Source: three-view drawing plus pictorial views. Frame: mm from the lowest corner of the part. A direction names the side the tool comes from. Give positions to 0.01 mm unless a question says otherwise; leave off trailing zeros. Write each loop counter-clockwise with the first axis right and the second up, starting at its lowest first coordinate (ties: lowest second). Pieces come first, ordered by that corner, then holes. Notation, with made-up numbers: M 57.5,29.25 L 66.5,29.25 A23 ccw 66.5,41.25 Z; hole C -13.75,11 d7. An arc over 180 degrees is marked long. One line per question, with ' | ' between items.
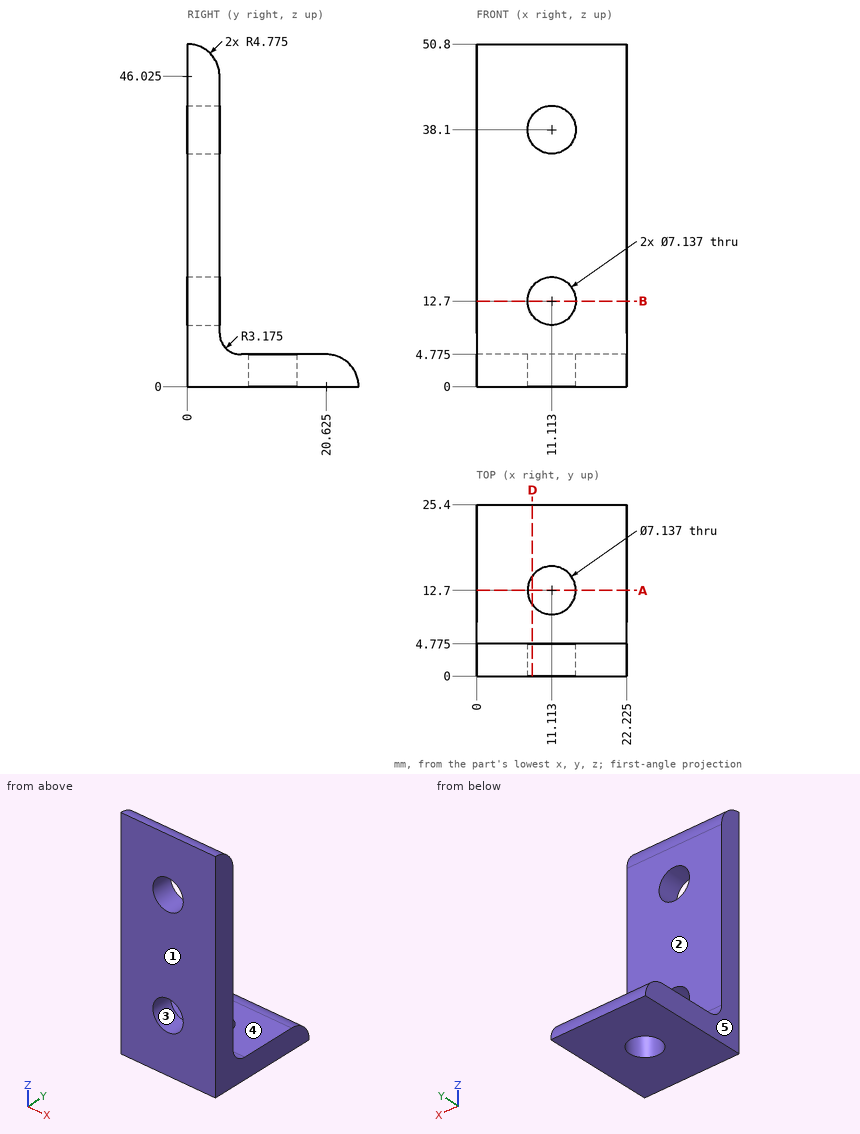
(1) Cut plane D-D, the plane x = 8.25. Count the separate pieces of the cut face and the enclosed holes in it.
Working result:
separate pieces: 4 | enclosed holes: 0
(2) Draft query along X for the marked faces 3, 4 and 5. Return one class per face: released by +X, released by -X, zero draft, split by the parting line, or undercut.
Working result:
face 3: undercut | face 4: zero draft | face 5: released by -X
(3) Set-up query: the marked faces 1 and 2. Return all of +Z, -Z, +X, -X, +Y, -Y with unobstructed straight access to the full face (end or side cutting, diameter ignored); none if empty.
Working result:
face 1: +Z, -Z, +X, -X, -Y | face 2: +Z, +X, -X, +Y
(4) Cut plane A-A, the plane y = 12.7. Return loops of the section in (x, z) (1 decimal).
Working result:
outline: M 0,0 L 7.5,0 L 7.5,4.8 L 0,4.8 Z; M 14.7,0 L 22.2,0 L 22.2,4.8 L 14.7,4.8 Z
(5) First-contact query: P1, Ø6, axis at x = 10, y = 12.5, coming from the +Z side (1 decimal); P2, Ø6, axis at x = 15.5, y = 5.5, coming from the +Z side. Flat tips, straight axial feed; report the tip coordinate or a pass-through.
Working result:
P1: stops at z = 4.8 | P2: stops at z = 50.09
(6) Material intervals for L1, parallel to X at y = 2.55, z = 12.7 (1 decimal); L2, parallel to Z at x = 8.75, y = 19 (1 decimal), sorted ascending. Write a range as [from, to].
Working result:
L1: x = [0, 7.5], [14.7, 22.2] | L2: z = [0, 4.8]
